Design review of the part built by this model. Coordinates are the model's own, in mm. Face numbers are marked on the shaded views. A direction names the side the tool comes from. Round coordinates to 2 decimals unless told otherwise and drop trailing zeros. Loops run counter-clockwise (first coordinate to the right, second up) from the corner with the lowest first, then second, coordinate; pieces in that order, holes last. Notation, with made-up numbers: (53.5, 35) -> (76.5, 35) arc R28 cw to (76.5, 69) -> close; hole circle Ø5 at (40.25, 32.25). An arc over 180 degrees is marked (long way). Use a Markdown table: item, result. Add a question column.
Autodesk Fusion 360 part; units mm, degrees
sketch "Sketch1" plane through (0, 0, 0) normal (0, 0, 1) x (1, 0, 0)
  line L0 (0, 0) -> (56.6, 0)
  line L1 (56.6, 0) -> (56.6, 30.7)
  line L2 (56.6, 30.7) -> (0, 30.7)
  line L3 (0, 30.7) -> (0, 0)
  dimension "d1" = 56.6
  dimension "d2" = 30.7
extrude "Extrude1" add sketch "Sketch1" along normal blind 14.4
sketch "Sketch2" plane through (0, 0, 0) normal (-1, 0, 0) x (0, -1, 0)
  line L0 (-30.7, 0) -> (0, 0)
  line L1 (0, 14.4) -> (-30.7, 14.4)
  line L2 (-30.7, 14.4) -> (-30.7, 0)
  line L3 (4.8, 12.6) -> (-3.2, 12.6)
  line L4 (-3.2, 12.6) -> (-3.2, 1.8)
  line L5 (-3.2, 1.8) -> (4.8, 1.8)
  line L6 (4.8, 1.8) -> (4.8, 12.6)
  line L7 (0, 0) -> (0, 14.4)
  dimension "d9" = 8
  dimension "d10" = 3.2
  dimension "d11" = 1.8
  dimension "d12" = 1.8
extrude "Extrude2" add sketch "Sketch2" along normal blind 10 contours L3 L5 L6 L7 | L3 L4 L5 L7
chamfer "Chamfer1" distance 4.8 angle 60 1 edges at (0, 0, 7.2) measured on face at (0, -1.6, 5.4)
equation "d12 = d11"
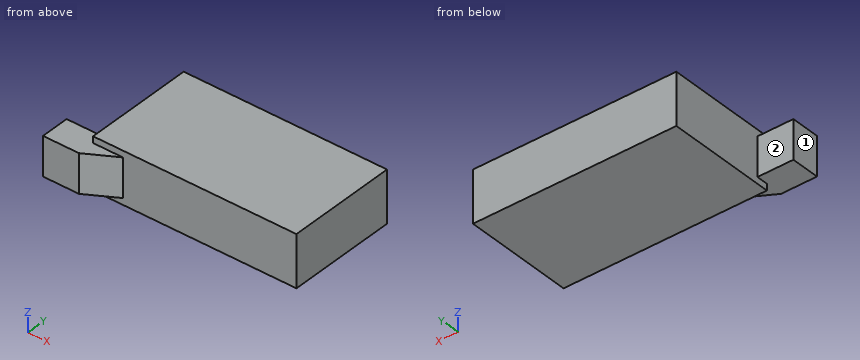
1. Consider section D-D on x = 27. State the section outline as (y, z) points.
2. For the marked faces 1 and 2, list the 3-axis set-ups (+Z, -Z, +X, -X, +Y, -Y) from which the entire face can be reached by the end or side of a thin tool; tool diameter is ignored.
3. Consider section B-B on x = 4.5. State the section outline as (y, z) points.
4. To check wall thickness, follow probe 1 along X at (y, z) = (29, 10); probe 2 along Y at (x, z) = (42, 7.75); probe 3 along Z at (x, y) = (-6, -2). State the ranges of each line that lie inside material, in increasing order. Write a range as from..to.
5. Consider section C-C on y = 21. State the section outline as (x, z) points.
6. Insertion check: P1, Ø3, axis at y = 7, z = 11.5, coming from the -X side; P2, Ø6, axis at x = 27, z = 9.5, coming from the -Y side. Each pin has a flat end and moves straight along its axis. Give the tip position at first contact, or say it passes through.
Verdict:
| question | item | result |
|---|---|---|
| 1 | outline | (0, 0) -> (30.7, 0) -> (30.7, 14.4) -> (0, 14.4) -> close |
| 2 | face 1 | +Z, -Z, -X, +Y, -Y |
| 2 | face 2 | +Z, -Z, -X, +Y |
| 3 | outline | (-2.2, 1.8) -> (0, 1.8) -> (0, 0) -> (30.7, 0) -> (30.7, 14.4) -> (0, 14.4) -> (0, 12.6) -> (-2.2, 12.6) -> close |
| 4 | probe 1 | x = 0..56.6 |
| 4 | probe 2 | y = 0..30.7 |
| 4 | probe 3 | z = 1.8..12.6 |
| 5 | outline | (0, 0) -> (56.6, 0) -> (56.6, 14.4) -> (0, 14.4) -> close |
| 6 | P1 | stops at x = 0 |
| 6 | P2 | stops at y = 0 |
